Input: part model. Units: mm. Frame: model coordinates. Face numbers are marked on the shaded views. Coordinates: 2 decimals unless noted, no trailing zeros. Loops run counter-clockwise (first coordinate to the right, second up) from the corner with the lowest first, then second, coordinate; pieces in that order, holes last. Notation, with made-up numbers: M -10.75,-39.5 L 36.25,-39.5 A25 cw 36.25,-4.5 Z; hole C -32,17.5 d10. An arc over 180 degrees is marked long. Use a Markdown table: item, result. Add a question column.
1. Section D-D on x = -14.5. Output: boundary loops of the cut face in (y, z), then the cut area to 3 significant figures.
2. Pin query (flat end, axial travel): pin 1 (16 mm diameter, centred on x = 0, z = -39.5, fed in from +Y); pin 2 (1 mm diameter, centred on x = -3, z = -62, fed in from -Y); pin 3 (10 mm diameter, centred on x = 11.5, z = -29, fed in from -Y). Return the tip coordinate at first contact, or that it passes through.
3. Section B-B on y = -4. Output: boundary loops of the cut face in (x, z), then the cut area to 3 significant figures.
4. Draft query along Z for the marked faces 1, 2 and 3. Return one class per face: +Z half, -Z half, draft (parallel to the pull), parting line (faces both ways), or undercut.
5. Section C-C on y = 11. Output: boundary loops of the cut face in (x, z), then the cut area to 3 significant figures.
6. Section A-A on x = 0. Output: boundary loops of the cut face in (y, z), then the cut area to 3 significant figures.
7. Line query: L1, parallel to X at y = 0, z = -48; L2, parallel to Y at x = 10.5, z = -14.5; L3, parallel to X at y = -11, z = -43.5. Output: solid intervals per line, ascending. Write a range as [from, to].
```python
from build123d import *

# Parameters (mm, degrees)
SKETCH1_R                = 17.5
SKETCH1_R_2              = 13.5
BOSS_EXTRUDE2_DEPTH      = 25
BOSS_EXTRUDE2_DEPTH_BACK = 17
SKETCH2_R                = 17.5
SKETCH3_R                = 13.5
CUT_EXTRUDE1_DEPTH       = 92.39748364
CUT_EXTRUDE2_REACH       = 102.734
CUT_EXTRUDE2_END_RADIUS  = 13.5
SKETCH4_R                = 13.5


with BuildPart() as part:
    # Sweep1: sweep along a curve in space
    with BuildLine() as sweep1_path:
        Line((0, 0, 0), (0, 0, -79))
    # Sketch1 → Sweep1 (sweep)
    with BuildSketch(Plane.XY):
        Circle(SKETCH1_R)
        Circle(SKETCH1_R_2, mode=Mode.SUBTRACT)
    sweep(path=sweep1_path.line)

    # Sketch2 → Boss-Extrude2 (add, two sides: drawn at the far end of the back side and taken through both)
    with BuildSketch(Plane(origin=(0, 17.5, 0), x_dir=(1, 0, 0), z_dir=(0, 1, 0)).offset(-BOSS_EXTRUDE2_DEPTH_BACK)):
        with Locations(Location((0, 39.5, 0), (0, 0, 270))):
            Circle(SKETCH2_R)
    extrude(amount=BOSS_EXTRUDE2_DEPTH + BOSS_EXTRUDE2_DEPTH_BACK)

    # Sketch3 → Cut-Extrude1 (cut, through all)
    with BuildSketch(Plane.XY):
        Circle(SKETCH3_R)
    extrude(amount=-CUT_EXTRUDE1_DEPTH, mode=Mode.SUBTRACT)

    # Cut-Extrude2: up to this cylinder (the profile starts outside it)
    cut_extrude2_end = Plane(origin=(0, 0, -39.5), z_dir=(0, 0, -1)) * Cylinder(CUT_EXTRUDE2_END_RADIUS, 233.468, mode=Mode.PRIVATE)
    # Sketch4 → Cut-Extrude2 (cut, up to the surface)
    with BuildSketch(Plane(origin=(0, 42.5, 0), x_dir=(1, 0, 0), z_dir=(0, 1, 0)), mode=Mode.PRIVATE) as cut_extrude2_sk1:
        with Locations(Location((0, 39.5, 0), (0, 0, 270))):
            Circle(SKETCH4_R)
    cut_extrude2_tool1 = extrude(cut_extrude2_sk1.sketch, amount=-CUT_EXTRUDE2_REACH, mode=Mode.PRIVATE) - cut_extrude2_end
    add(cut_extrude2_tool1.solids().sort_by_distance((0, 42.5, -39.5))[0], mode=Mode.SUBTRACT)


solid = part.part
```
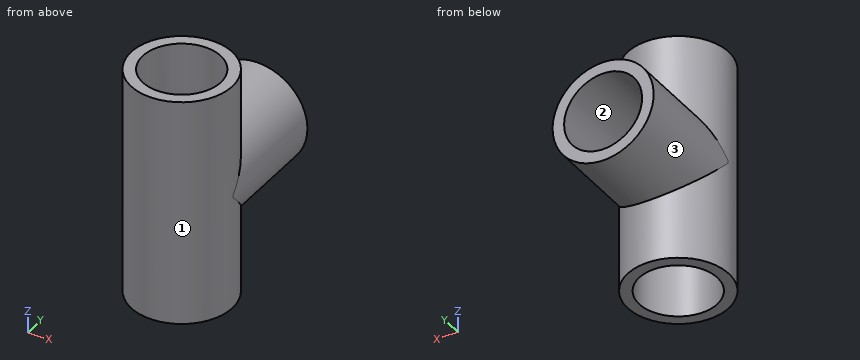
Answers below:
| question | item | result |
|---|---|---|
| 1 | outline | M -9.8,-79 L 9.8,-79 L 9.8,-49.3 L 42.5,-49.3 L 42.5,-29.7 L 9.8,-29.7 L 9.8,0 L -9.8,0 Z |
| 1 | area | 2,190 mm² |
| 2 | pin 1 | stops at y = -10.87 |
| 2 | pin 2 | stops at y = -17.32 |
| 2 | pin 3 | stops at y = -16.25 |
| 3 | outline | M -17.04,-79 L -12.89,-79 L -12.89,0 L -17.04,0 Z; M 12.89,-79 L 17.04,-79 L 17.04,0 L 12.89,0 Z |
| 3 | area | 655 mm² |
| 4 | face 1 | draft |
| 4 | face 2 | undercut |
| 4 | face 3 | parting line |
| 5 | outline | M -13.61,-79 L -7.83,-79 L -7.83,-50.5 A13.5 cw -7.83,-28.5 L -7.83,0 L -13.61,0 L -13.61,-28.5 A17.5 ccw -13.61,-50.5 Z; M 7.83,-79 L 13.61,-79 L 13.61,-50.5 A17.5 ccw 13.61,-28.5 L 13.61,0 L 7.83,0 L 7.83,-28.5 A13.5 cw 7.83,-50.5 Z |
| 5 | area | 856 mm² |
| 6 | outline | M -17.5,-79 L -13.5,-79 L -13.5,0 L -17.5,0 Z; M 13.5,-79 L 17.5,-79 L 17.5,-57 L 42.5,-57 L 42.5,-53 L 13.5,-53 Z; M 13.5,-26 L 42.5,-26 L 42.5,-22 L 17.5,-22 L 17.5,0 L 13.5,0 Z |
| 6 | area | 724 mm² |
| 7 | L1 | x = [-17.5, -13.5], [13.5, 17.5] |
| 7 | L2 | y = [-14, -8.49], [8.49, 14] |
| 7 | L3 | x = [-13.61, -7.83], [7.83, 13.61] |
